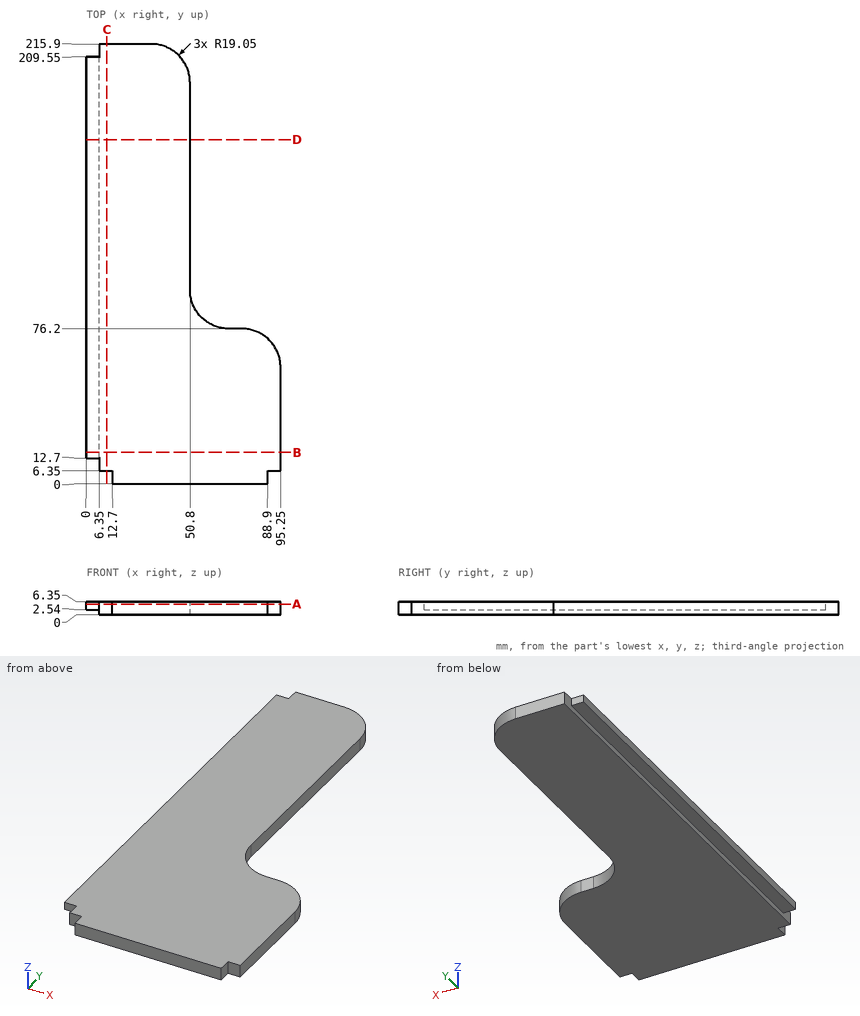
Job drawing, mm, ordinate dimensions from the low corner. One solid piece. Round coordinates to 2 decimals unless told otherwise and drop trailing zeros. Write each loop counter-clockwise with the first axis right and the second up, starting at its lowest first coordinate (ties: lowest second). Pieces come first, ordered by that corner, then holes.
1) Band-saw the part on A-A, the plane z = 5.25. List the corners of the cut face in (x, y).
2) Drill centre lines: probe 1 along X at (y, z) = (144.5, 6); probe 2 along X at (y, z) = (133.5, 0.75); probe 3 along Y at (x, z) = (91, 3.25). Where is each one in solid material? Low to high.
3) Pin check, flat tips, straight feed: pin 1 (3 mm diameter, centred on x = 9, z = 1.5, fed in from -Y); pin 2 (3 mm diameter, centred on y = 1.5, z = 4, fed in from -X); pin 3 (5 mm diameter, centred on x = 51, y = 147.5, fed in from +Z); pin 4 (3 mm diameter, centred on y = 2, z = 2, fed in from +X). Stop position of each tip, or through.
4) Band-saw the part on D-D, the plane y = 169. List the corners of the cut face in (x, z).
5) Band-saw the part on B-B, the plane y = 15.5. List the corners of the cut face in (x, z), and give its area (3 significant figures).
6) Band-saw the part on C-C, the plane x = 10. List the corners of the cut face in (y, z), and give its area (3 significant figures).
Ans:
1. outline: (0, 12.7) - (6.35, 12.7) - (6.35, 6.35) - (12.7, 6.35) - (12.7, 0) - (88.9, 0) - (88.9, 6.35) - (95.25, 6.35) - (95.25, 57.15) arc R19.05 ccw to (76.2, 76.2) - (69.85, 76.2) arc R19.05 cw to (50.8, 95.25) - (50.8, 196.85) arc R19.05 ccw to (31.75, 215.9) - (6.35, 215.9) - (6.35, 209.55) - (0, 209.55) - close
2. probe 1: x = 0 to 50.8
2. probe 2: x = 6.35 to 50.8
2. probe 3: y = 6.35 to 69.14
3. pin 1: stops at y = 6.35
3. pin 2: stops at x = 12.7
3. pin 3: stops at z = 6.35
3. pin 4: stops at x = 88.9
4. outline: (0, 2.54) - (6.35, 2.54) - (6.35, 0) - (50.8, 0) - (50.8, 6.35) - (0, 6.35) - close
5. outline: (0, 2.54) - (6.35, 2.54) - (6.35, 0) - (95.25, 0) - (95.25, 6.35) - (0, 6.35) - close
5. area: 589 mm2
6. outline: (6.35, 0) - (215.9, 0) - (215.9, 6.35) - (6.35, 6.35) - close
6. area: 1,330 mm2
